For this review, take the finished solid that the model builds, in its own axes (mm). A direction names the side the tool comes from. Round coordinates to 2 decimals unless told otherwise and drop trailing zeros. Order: outer loops, then holes, each group sorted by start corner. A loop starts at its lowest first (then second) coordinate and runs counter-clockwise, first axis right, second up. Notation, with made-up numbers: (-4.75, 33.5) -> (19.25, 33.5) arc R29 cw to (19.25, 71.5) -> close; hole circle Ø11 at (-29.75, -24.75). An arc over 180 degrees is marked (long way). Use a Markdown table: item, result. Add a question column.
1) Clearance check with flat-ended pins moving along their axes: P1, Ø10, axis at x = 25, z = -2, coming from the +Y side (3 decimals); P2, Ø7, axis at y = 0.5, z = -1, coming from the +X side (3 decimals). State where each tip first meets the part, or that it passes through.
2) Consider section C-C (y = -4). State the section outline as (x, z) points (3 decimals), plus the area to 3 significant figures.
3) Consider section A-A (x = 14). State the section outline as (y, z) points (3 decimals).
4) Machinability: for faces 1 (the face through (0.13, 27.69, 7.31)), 2 (the face through (20.542, -11.053, -8.076)), 3 (the face through (39.747, -18.988, -8.076)), 4 (the face through (23, -9.525, 0)), 5 (the face through (20.542, -10.974, 7.997)), which of the approach directions +Z, -Z, +X, -X, +Y, -Y give a long, thin tool a straight path to every point of the face, cutting with its end or side? Answer none if there is none.
5) Consider section D-D (x = -2). State the section outline as (y, z) points (3 decimals).
6) Wall thickness on line 1 along Y through (x, z) = (24.5, -4.5); line 2 along X through (y, z) = (2, 2.5) (3 decimals); line 3 along Y through (x, z) = (27.5, 5.5): over which ranges is each line inside the solid? List them lowest first. Write a range as [from, to].
7) Consider section B-B (z = 1.5). State the section outline as (x, y) points (3 decimals), plus the area to 3 significant figures.
```python
from build123d import *

# Parameters (mm, degrees)
F0_W     = 19.05
F0_H     = 57.15
F1_DEPTH = 9.525
F2_W     = 19.05
F2_H     = 19.05
F3_DEPTH = 31.75
F4_R     = 5.08


with BuildPart() as f1:
    # F0 (on Top) → F1 (new body, symmetric)
    with BuildSketch(Plane.XY):
        Rectangle(F0_W, F0_H)
    extrude(amount=F1_DEPTH, both=True)

    # F2 (on face) → F3 (join)
    with BuildSketch(Plane.YZ.offset(9.525)):
        with Locations((-19.05, 0)):
            Rectangle(F2_W, F2_H)
    extrude(amount=F3_DEPTH)

    # F4
    f4_edges = [f1.edges().sort_by_distance(p)[0] for p in [
        (9.525, 9.525, 9.525),
        (15.875, -28.575, 9.525),
        (41.275, -19.05, 9.525),
        (25.4, -9.525, 9.525),
        (0, 28.575, 9.525),
        (-9.525, 0, 9.525),
        (15.875, -28.575, -9.525),
        (41.275, -28.575, 0),
        (41.275, -9.525, 0),
        (41.275, -19.05, -9.525),
        (-9.525, 0, -9.525),
        (-9.525, -28.575, 0),
        (9.525, 9.525, -9.525),
        (25.4, -9.525, -9.525),
    ]]
    fillet(f4_edges, radius=F4_R)


solid = f1.part
```
Results list:
| question | item | result |
|---|---|---|
| 1 | P1 | y = -9.525 |
| 1 | P2 | x = 9.525 |
| 2 | outline | (-9.525, -4.445) arc R5.08 ccw to (-4.445, -9.525) -> (4.445, -9.525) arc R5.08 ccw to (9.525, -4.445) -> (9.525, 4.445) arc R5.08 ccw to (4.445, 9.525) -> (-4.445, 9.525) arc R5.08 ccw to (-9.525, 4.445) -> close |
| 2 | area | 341 mm2 |
| 3 | outline | (-28.575, -4.445) arc R5.08 ccw to (-23.495, -9.525) -> (-14.605, -9.525) arc R5.08 ccw to (-9.525, -4.445) -> (-9.525, 4.445) arc R5.08 ccw to (-14.605, 9.525) -> (-23.495, 9.525) arc R5.08 ccw to (-28.575, 4.445) -> close |
| 4 | face 1 | +Z, +X, -X, +Y |
| 4 | face 2 | -Z, +X, +Y |
| 4 | face 3 | -Z, +X, +Y, -Y |
| 4 | face 4 | +Z, -Z, +X, +Y |
| 4 | face 5 | +Z, +X, +Y |
| 5 | outline | (-28.575, -4.445) arc R5.08 ccw to (-23.495, -9.525) -> (28.575, -9.525) -> (28.575, 4.445) arc R5.08 ccw to (23.495, 9.525) -> (-23.495, 9.525) arc R5.08 ccw to (-28.575, 4.445) -> close |
| 6 | line 1 | [-28.57, -9.53] |
| 6 | line 2 | [-9.525, 9.525] |
| 6 | line 3 | [-28.46, -9.64] |
| 7 | outline | (-9.525, -23.495) arc R5.08 ccw to (-4.445, -28.575) -> (36.195, -28.575) arc R5.08 ccw to (41.275, -23.495) -> (41.275, -14.605) arc R5.08 ccw to (36.195, -9.525) -> (9.525, -9.525) -> (9.525, 28.575) -> (-9.525, 28.575) -> close |
| 7 | area | 1,680 mm2 |
